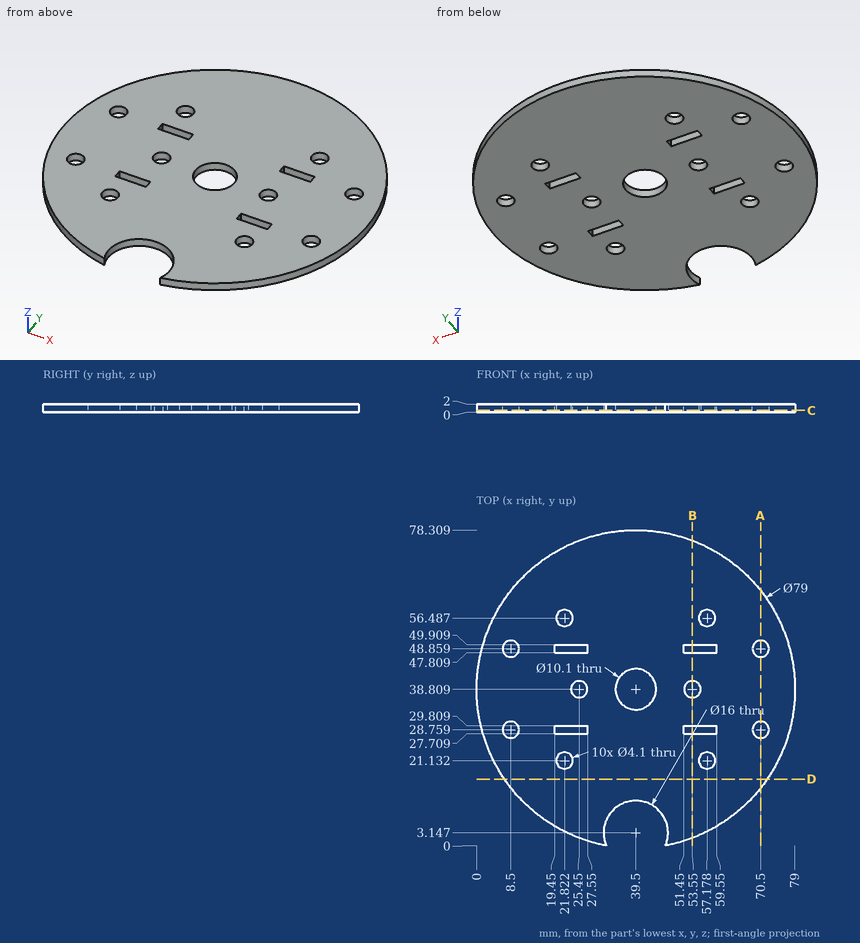
Check sheet for the drawn part. Datum: minimum x, y, z corner. Units: mm. Round coordinates to 2 decimals unless told otherwise and drop trailing zeros. Order: outer loops, then holes, each group sorted by start corner. A loop starts at its lowest first (then second) coordinate and runs counter-clockwise, first axis right, second up.
(1) Go/stop test with flat-tipped pins: P1, Ø2.5, axis at x = 70.5, y = 28.76, coming from the -Z side; P2, Ø2, axis at x = 39.5, y = 49, coming from the -Z side; P3, Ø1, axis at x = 54.5, z = 1, coming from the -Y side; P4, Ø0.6, axis at y = 49, z = 1, coming from the -X side. Record where each tip stops, or that it passes through.
(2) Cross-section at D-D, the plane y = 16.5. Enter the section's corners in (x, z).
(3) Cross-section at C-C, the plane z = 0.4. State how many separate pieces and enclosed holes the cut face has.
(4) Scan lines: probe 1 along X at (y, z) = (19.5, 1.15) (1 decimal); probe 2 along Y at (x, z) = (8.5, 0.8); probe 3 along X at (y, z) = (50, 1.9) (1 decimal). Record each from-to range of solid material in increasing order.
(5) Cross-section at B-B, the plane x = 53.55. Enter the section's corners in (y, z), and give its area (3 significant figures).
(6) Cross-section at A-A, the plane x = 70.5. Enter the section's corners in (y, z).
Check sheet entries:
1. P1: passes through
1. P2: stops at z = 0
1. P3: stops at y = 2.07
1. P4: stops at x = 1.26
2. outline: (6.9, 0) - (72.1, 0) - (72.1, 2) - (6.9, 2) - close
3. separate pieces: 1
3. enclosed holes: 15
4. probe 1: x = 5 to 20.6, 23.1 to 55.9, 58.4 to 74
4. probe 2: y = 14.33 to 26.71, 30.81 to 46.81, 50.91 to 63.29
4. probe 3: x = 1.6 to 6.8, 10.2 to 68.8, 72.2 to 77.4
5. outline: (1.89, 0) - (27.71, 0) - (27.71, 2) - (1.89, 2) - close; (29.81, 0) - (36.76, 0) - (36.76, 2) - (29.81, 2) - close; (40.86, 0) - (47.81, 0) - (47.81, 2) - (40.86, 2) - close; (49.91, 0) - (75.73, 0) - (75.73, 2) - (49.91, 2) - close
5. area: 131 mm2
6. outline: (14.33, 0) - (26.71, 0) - (26.71, 2) - (14.33, 2) - close; (30.81, 0) - (46.81, 0) - (46.81, 2) - (30.81, 2) - close; (50.91, 0) - (63.29, 0) - (63.29, 2) - (50.91, 2) - close
